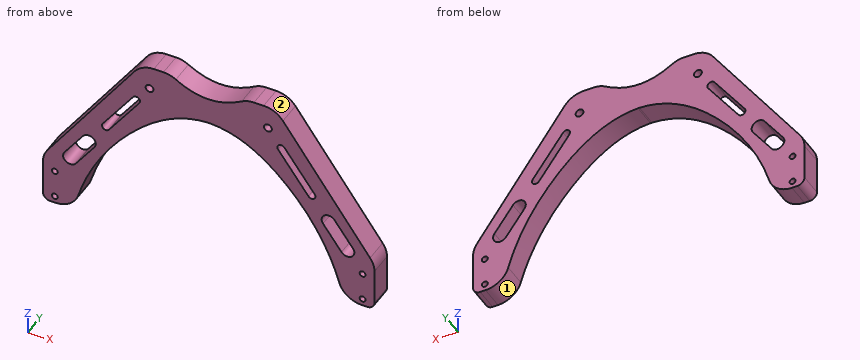
```python
from build123d import *

# Parameters (mm, degrees)
SKETCH_1_W          = 140
SKETCH_1_H          = 80
SKETCH_1_R          = 1.25
SKETCH_1_R_2        = 1.65
EXTRUDE_1_DEPTH     = 10
CUT_EXTRUDE_1_DEPTH = 101.204790305
FILLET_1_R          = 10
FILLET_2_R          = 3
CUT_EXTRUDE_2_DEPTH = 101.204790455


with BuildPart() as part:
    # 草图1 → 凸台-拉伸1 (new body)
    with BuildSketch(Plane(origin=(0, 0, 0), x_dir=(1, 0, 0), z_dir=(0, 1, 0))):
        with Locations((0, -31)):
            Rectangle(SKETCH_1_W, SKETCH_1_H)
        with Locations(Location((-65, 6, 0), (0, 0, 270))):
            Circle(SKETCH_1_R, mode=Mode.SUBTRACT)
        with Locations(Location((-65, -6, 0), (0, 0, 270))):
            Circle(SKETCH_1_R, mode=Mode.SUBTRACT)
        with Locations(Location((65, -6, 0), (0, 0, 90))):
            Circle(SKETCH_1_R, mode=Mode.SUBTRACT)
        with Locations(Location((65, 6, 0), (0, 0, 90))):
            Circle(SKETCH_1_R, mode=Mode.SUBTRACT)
        with Locations(Location((-25, -61, 0), (0, 0, 270))):
            Circle(SKETCH_1_R_2, mode=Mode.SUBTRACT)
        with Locations(Location((25, -61, 0), (0, 0, 90))):
            Circle(SKETCH_1_R_2, mode=Mode.SUBTRACT)
    extrude(amount=EXTRUDE_1_DEPTH)

    # 草图2 → 切除-拉伸1 (cut, through all)
    with BuildSketch(Plane(origin=(0, 10, 0), x_dir=(1, 0, 0), z_dir=(0, 1, 0))):
        Polygon((-70, -12.331865366), (-28.346020761, -71), (-70, -71), align=None)
        Polygon((70, -12.331865366), (28.346020761, -71), (70, -71), align=None)
        with BuildLine():
            Line((-16.105693614, -71), (16.105693614, -71))
            add(Edge.make_bspline(
                [(-16.105693614, -71), (0, -59.46206609), (16.105693614, -71)],
                knots=[0, 0, 0, 1, 1, 1], degree=2))
        make_face()
        with BuildLine():
            Line((56.906784104, 9), (-56.906784104, 9))
            add(Edge.make_bspline(
                [(-56.906784104, 9), (-53.268076424, -8.599244087), (-38.630052836, -35.640481439), (-12.875691634, -53.653343186), (0, -53.936278292)],
                knots=[0, 0, 0, 0, 0.590583246, 1, 1, 1, 1], degree=3))
            add(Edge.make_bspline(
                [(56.906784104, 9), (53.268076424, -8.599244087), (38.630052836, -35.640481439), (12.875691634, -53.653343186), (0, -53.936278292)],
                knots=[0, 0, 0, 0, 0.590583246, 1, 1, 1, 1], degree=3))
        make_face()
    extrude(amount=-CUT_EXTRUDE_1_DEPTH, mode=Mode.SUBTRACT)

    # 圆角1
    # the kernel refuses this fillet: 10 mm, written as the material it adds along each edge
    with BuildSketch(Plane(origin=(0, 10, 53.936278292), x_dir=(-0.999651568741567, 0, -0.026395854078324985), z_dir=(0, -1, 0))) as fillet_1_piece_1:
        with BuildLine():
            CenterArc((0.264047953, 9.999901848), FILLET_1_R, 266.721049901, 3.532806773)
            Line((-0.307924469, 0.016272871), (-0.319363918, -0.183399709))
            ThreePointArc((-0.319363918, -0.183399709), (-0.16453479, -0.191925855), (-0.009670177, -0.199766082))
            Line((-0.009670177, -0.199766082), (-0.000885616, -0.199998039))
            ThreePointArc((-0.000885616, -0.199998039), (0.15417695, -0.200341456), (0.30924028, -0.199998037))
            Line((0.30924028, -0.199998037), (0.308354155, 0))
        make_face()
    extrude(amount=10)
    # the kernel refuses this fillet: 10 mm, written as the material it takes off along each edge
    with BuildSketch(Plane(origin=(-70, 10, 12.331865366), x_dir=(0.5789182566890616, 0, 0.8153855849057535), z_dir=(0, -1, 0)), Plane(origin=(70, 10, 12.331865366), x_dir=(0, 0, -1), z_dir=(0, -1, 0))) as fillet_1_2_piece_1:
        with BuildLine():
            CenterArc((FILLET_1_R * 0.318895479562, -FILLET_1_R), FILLET_1_R, 90, 35.374494493)
            Line((-FILLET_1_R * 0.260022777127, -FILLET_1_R * 0.184614415094), (-FILLET_1_R * 0.271601142261, -FILLET_1_R * 0.168306703396))
            Line((-FILLET_1_R * 0.271601142261, -FILLET_1_R * 0.168306703396), (-FILLET_1_R * 0.00637790959125, FILLET_1_R * 0.02))
            Line((-FILLET_1_R * 0.00637790959125, FILLET_1_R * 0.02), (FILLET_1_R * 0.318895479562, FILLET_1_R * 0.02))
            Line((FILLET_1_R * 0.318895479562, FILLET_1_R * 0.02), (FILLET_1_R * 0.318895479562, 0))
        make_face()
    extrude(amount=10, mode=Mode.SUBTRACT)
    with BuildSketch(Plane(origin=(-56.906784104, 10, -9), x_dir=(-1, 0, 0), z_dir=(0, -1, 0))) as fillet_1_2_piece_2:
        with BuildLine():
            CenterArc((7.807317394, -10), FILLET_1_R, 90, 73.718330192)
            Line((-1.79163295, -7.196403685), (-1.983611957, -7.140331758))
            ThreePointArc((-1.983611957, -7.140331758), (-1.017653275, -3.56787057), (-0.195857636, 0.040494278))
            Line((-0.195857636, 0.040494278), (0, 0.2))
            Line((0, 0.2), (7.807317394, 0.2))
            Line((7.807317394, 0.2), (7.807317394, 0))
        make_face()
    extrude(amount=10, mode=Mode.SUBTRACT)
    with BuildSketch(Plane(origin=(56.906784104, 10, -9), x_dir=(-0.2415877467248244, 0, 0.9703789778392884), z_dir=(0, -1, 0))) as fillet_1_2_piece_3:
        with BuildLine():
            CenterArc((7.817637561, -9.991934139), FILLET_1_R, 92.301400389, 73.718330192)
            Line((-1.886152217, -7.576056672), (-2.080228013, -7.527739123))
            Line((-2.080228013, -7.527739123), (-0.194075796, 0.048317549))
            Line((-0.194075796, 0.048317549), (0.008022009, 0.199839054))
            ThreePointArc((0.008022009, 0.199839054), (3.708039158, 0.125555533), (7.408044176, 0.199838683))
            Line((7.408044176, 0.199838683), (7.416075419, 0))
        make_face()
    extrude(amount=10, mode=Mode.SUBTRACT)
    with BuildSketch(Plane(origin=(-28.346020761, 10, 71), x_dir=(1, 0, 0), z_dir=(0, -1, 0)), Plane(origin=(28.346020761, 10, 71), x_dir=(0.5789182566890612, 0, -0.8153855849057537), z_dir=(0, -1, 0))) as fillet_1_2_piece_4:
        with BuildLine():
            CenterArc((FILLET_1_R * 0.516420391905, -FILLET_1_R), FILLET_1_R, 90, 54.625505507)
            Line((-FILLET_1_R * 0.298965193, -FILLET_1_R * 0.421081743311), (-FILLET_1_R * 0.315272904699, -FILLET_1_R * 0.409503378177))
            Line((-FILLET_1_R * 0.315272904699, -FILLET_1_R * 0.409503378177), (-FILLET_1_R * 0.0103284078381, FILLET_1_R * 0.02))
            Line((-FILLET_1_R * 0.0103284078381, FILLET_1_R * 0.02), (FILLET_1_R * 0.516420391905, FILLET_1_R * 0.02))
            Line((FILLET_1_R * 0.516420391905, FILLET_1_R * 0.02), (FILLET_1_R * 0.516420391905, 0))
        make_face()
    extrude(amount=10, mode=Mode.SUBTRACT)
    with BuildSketch(Plane(origin=(-16.105693614, 10, 71), x_dir=(-1, 0, 0), z_dir=(0, -1, 0))) as fillet_1_2_piece_5:
        with BuildLine():
            CenterArc((3.016711089, 10), FILLET_1_R, 238.325124011, 31.674875989)
            Line((-2.234274138, 1.489585548), (-2.339293843, 1.319377259))
            ThreePointArc((-2.339293843, 1.319377259), (-1.215329893, 0.597636236), (-0.116473908, -0.162584835))
            Line((-0.116473908, -0.162584835), (0, -0.2))
            Line((0, -0.2), (3.016711089, -0.2))
            Line((3.016711089, -0.2), (3.016711089, 0))
        make_face()
    extrude(amount=10, mode=Mode.SUBTRACT)
    with BuildSketch(Plane(origin=(16.105693614, 10, 71), x_dir=(-0.8320383563974485, 0, -0.554718102718338), z_dir=(0, -1, 0))) as fillet_1_2_piece_6:
        with BuildLine():
            CenterArc((3.037161691, 9.993807815), FILLET_1_R, 236.308699407, 31.674875989)
            Line((-2.510019336, 1.673424251), (-2.620962956, 1.50701658))
            Line((-2.620962956, 1.50701658), (-0.110943621, -0.166407671))
            Line((-0.110943621, -0.166407671), (0.006722008, -0.199887005))
            ThreePointArc((0.006722008, -0.199887005), (1.342720726, -0.176909221), (2.678264654, -0.199876156))
            Line((2.678264654, -0.199876156), (2.685301851, 0))
        make_face()
    extrude(amount=10, mode=Mode.SUBTRACT)

    # 圆角2
    fillet_2_edges = [part.edges().sort_by_distance(p)[0] for p in [
        (-70, 5, -9),
        (70, 5, -9),
    ]]
    fillet(fillet_2_edges, radius=FILLET_2_R)

    # 草图3 → 切除-拉伸2 (cut, through all)
    with BuildSketch(Plane(origin=(0, 10, 0), x_dir=(1, 0, 0), z_dir=(0, 1, 0))):
        with BuildLine():
            Line((29.324357242, -52.277909179), (42.133187381, -34.665767738))
            ThreePointArc((42.133187381, -34.665767738), (44.414090847, -34.305625086), (44.774233499, -36.586528552))
            Line((44.774233499, -36.586528552), (31.965403361, -54.198669993))
            ThreePointArc((31.965403361, -54.198669993), (29.684499894, -54.558812645), (29.324357242, -52.277909179))
        make_face()
        with BuildLine():
            Line((60.93603818, -16.688498943), (53.122046102, -27.432738051))
            ThreePointArc((53.122046102, -27.432738051), (48.931322756, -28.09443121), (48.269629596, -23.903707865))
            Line((48.269629596, -23.903707865), (56.083621674, -13.159468757))
            ThreePointArc((56.083621674, -13.159468757), (60.27434502, -12.497775597), (60.93603818, -16.688498943))
        make_face()
        with BuildLine():
            Line((-60.93603818, -16.688498943), (-53.122046102, -27.432738051))
            ThreePointArc((-53.122046102, -27.432738051), (-48.931322756, -28.09443121), (-48.269629596, -23.903707865))
            Line((-48.269629596, -23.903707865), (-56.083621674, -13.159468757))
            ThreePointArc((-56.083621674, -13.159468757), (-60.27434502, -12.497775597), (-60.93603818, -16.688498943))
        make_face()
        with BuildLine():
            Line((-29.324357242, -52.277909179), (-42.133187381, -34.665767738))
            ThreePointArc((-42.133187381, -34.665767738), (-44.414090847, -34.305625086), (-44.774233499, -36.586528552))
            Line((-44.774233499, -36.586528552), (-31.965403361, -54.198669993))
            ThreePointArc((-31.965403361, -54.198669993), (-29.684499894, -54.558812645), (-29.324357242, -52.277909179))
        make_face()
    extrude(amount=-CUT_EXTRUDE_2_DEPTH, mode=Mode.SUBTRACT)


solid = part.part
```
The model under review builds one solid part; all positions refer to its coordinate system, in mm. Face numbers are marked on the shaded views. A direction names the side the tool comes from. Round coordinates to 2 decimals unless told otherwise and drop trailing zeros. Write each loop counter-clockwise with the first axis right and the second up, starting at its lowest first coordinate (ties: lowest second). Pieces come first, ordered by that corner, then holes.
(1) We need section A-A on z = 61. Give the boundary of the cut face in (x, y), and give its area (3 significant figures).
(2) We need section B-B on y = 7. Give the number of separate pieces and of enclosed holes in the cut face, and give its area (3 significant figures).
(3) Insertion check: pin 1 (1.5 mm diameter, centred on x = -6.5, y = 5, fed in from -Z); pin 2 (3 mm diameter, centred on x = -65, z = -6, fed in from +Y); pin 3 (4 mm diameter, centred on x = -51.5, y = 3, fed in from +Z). Each pin has a flat end and moves straight along its axis. Give the tip position at first contact, or say it passes through.
(4) Wall thickness on L1, parallel to X at y = 5, z = 43; L2, parallel to X at y = 9, z = 22; L3, parallel to X at y = 5.5, z = 2: over which ranges is each line inside the solid? List them lowest first.
(5) Machinability: for the marked faces 1 and 2, which of the approach directions +Z, -Z, +X, -X, +Y, -Y give a long, thin tool a straight path to every point of the face, cutting with its end or side? Answer none if there is none.
Findings below:
1. outline: (-35.45, 0) - (-26.65, 0) - (-26.65, 10) - (-35.45, 10) - close; (-23.35, 0) - (23.35, 0) - (23.35, 10) - (-23.35, 10) - close; (26.65, 0) - (35.45, 0) - (35.45, 10) - (26.65, 10) - close
1. area: 643 mm2
2. separate pieces: 1
2. enclosed holes: 10
2. area: 3,080 mm2
3. pin 1: stops at z = 53.01
3. pin 2: stops at y = 10
3. pin 3: stops at z = 41.21
4. L1: x = -48.23 to -40.11, -36.07 to -26.07, 26.07 to 36.07, 40.11 to 48.23
4. L2: x = -63.14 to -57.07, -49.65 to -44.31, 44.31 to 49.65, 57.07 to 63.14
4. L3: x = -70 to -53.91, 53.91 to 70
5. face 1: -Z, +Y, -Y
5. face 2: +Z, +X, +Y, -Y
